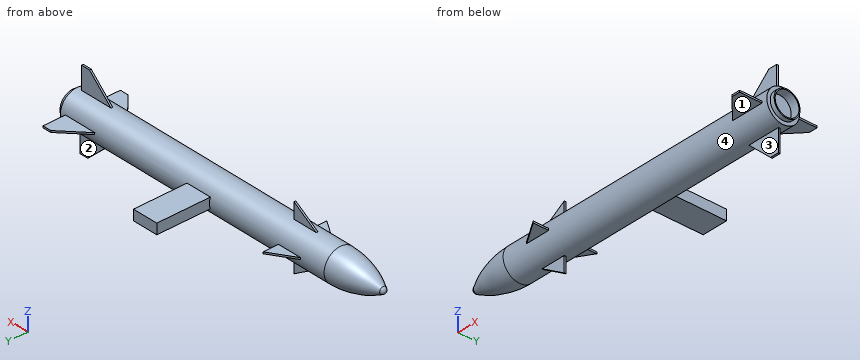
from build123d import *

# Parameters (mm, degrees)
D_ME1_FACE_RADIUS            = 400
D_ME1_HEIGHT                 = 290
ESQUISSE2_R                  = 1377.564968988
ENL_V_MAT_EXTRU_1_DEPTH      = 1000
BOSS_EXTRU_1_DEPTH           = 200
R_P_TITION_CIRCULAIRE1_COUNT = 4
BOSS_EXTRU_2_DEPTH           = 100
R_P_TITION_CIRCULAIRE2_COUNT = 4
ESQUISSE6_W                  = 3000
ESQUISSE6_H                  = 1200
BOSS_EXTRU_3_DEPTH           = 8000
ECHELLE1_SCALE               = 0.05


with BuildPart() as part:
    # Esquisse1 → Révolution1 (revolve)
    with BuildSketch(Plane(origin=(0, 0, 0), x_dir=(1, 0, 0), z_dir=(0, 1, 0))):
        with BuildLine():
            Line((0, 0), (0, 400))
            ThreePointArc((0, 400), (2649.561437252, 1518.274730075), (5500, 1900))
            Line((5500, 1900), (39500, 1900))
            Line((39500, 1900), (39500, 1500))
            Line((39500, 1500), (40000, 1500))
            Line((40000, 1500), (40000, 0))
            Line((40000, 0), (0, 0))
        make_face()
    revolve(axis=Axis((40000, 0, 0), (-1, 0, 0)))

    # Dôme1: a dome of height H over a round flat face of radius A is a cap of a sphere of radius (A * A + H * H) / (2 * H)
    d_me1_r = (D_ME1_FACE_RADIUS * D_ME1_FACE_RADIUS + D_ME1_HEIGHT * D_ME1_HEIGHT) / (2 * D_ME1_HEIGHT)
    d_me1_base = Plane((0, 0, 0), z_dir=(-1, 0, 0))
    with Locations(d_me1_base.offset(D_ME1_HEIGHT - d_me1_r)):
        d_me1_ball = Sphere(d_me1_r, mode=Mode.PRIVATE)
    add(split(d_me1_ball, bisect_by=d_me1_base, keep=Keep.TOP, mode=Mode.PRIVATE))

    # Esquisse2 → Enlèv. mat.-Extru.1 (cut)
    with BuildSketch(Plane(origin=(40000, 0, 0), x_dir=(0, 0, -1), z_dir=(1, 0, 0))):
        Circle(ESQUISSE2_R)
    extrude(amount=-ENL_V_MAT_EXTRU_1_DEPTH, mode=Mode.SUBTRACT)

    # Esquisse3 → Boss.-Extru.1 (add)
    with BuildSketch(Plane.XY):
        Polygon((38867.882175008, 1693.755150427), (38867.882175008, 4480.75805387), (37867.882175008, 4480.75805387), (34867.882175008, 1693.755150427), align=None)
    boss_extru_1 = extrude(amount=BOSS_EXTRU_1_DEPTH)

    # Répétition circulaire1: Boss.-Extru.1 ×4 about axis
    r_p_tition_circulaire1_axis = Axis((0, 0, 0), (1, 0, 0))
    for i in range(1, R_P_TITION_CIRCULAIRE1_COUNT):
        add(boss_extru_1.rotate(r_p_tition_circulaire1_axis, i * 360 / R_P_TITION_CIRCULAIRE1_COUNT))

    # Esquisse4 → Boss.-Extru.2 (add, symmetric)
    with BuildSketch(Plane.XY):
        Polygon((8155.279549148, 1665.288677311), (11371.991011305, 3686.408268577), (11371.991011305, 1665.288677311), align=None)
    boss_extru_2 = extrude(amount=BOSS_EXTRU_2_DEPTH, both=True)

    # Répétition circulaire2: Boss.-Extru.2 ×4 about axis
    r_p_tition_circulaire2_axis = Axis((0, 0, 0), (1, 0, 0))
    for i in range(1, R_P_TITION_CIRCULAIRE2_COUNT):
        add(boss_extru_2.rotate(r_p_tition_circulaire2_axis, i * 360 / R_P_TITION_CIRCULAIRE2_COUNT))

    # Esquisse6 → Boss.-Extru.3 (add)
    with BuildSketch(Plane(origin=(0, 0, 0), x_dir=(1, 0, 0), z_dir=(0, 1, 0))):
        with Locations((21779.89327035, -36.087335649)):
            Rectangle(ESQUISSE6_W, ESQUISSE6_H)
    extrude(amount=BOSS_EXTRU_3_DEPTH)


with BuildPart() as part_1:
    # Echelle1: scaled about (20884.167787821, 241.899239244, 1.78815963)
    add(part.part.scale(ECHELLE1_SCALE).moved(Location((19839.95939843, 229.804277282, 1.698751648))))


solid = part_1.part
Can you work these out from the model? Positions are in its coordinate system, mm. Face numbers are marked on the shaded views. A direction names the side the tool comes from. Give positions to 0.01 mm unless a question says otherwise; leave off trailing zeros. Loops run counter-clockwise (first coordinate to the right, second up) from the corner with the lowest first, then second, coordinate; pieces in that order, holes last. Notation, with made-up numbers: (16.25, 0.25) -> (55.25, 0.25) arc R11 ccw to (55.25, 13.25) -> close; hole circle Ø3 at (86, 11.25). An arc over 180 degrees is marked (long way). Return JSON: item names as keys, results as strings.
Q1. I want a section at A-A, the plane z = 145. List the corners of the cut face in (x, y) for me.
Checks:
{"outline": "(20343.27, 224.8) -> (20408.56, 224.8) -> (20408.56, 234.8) -> (20343.27, 234.8) -> close; (21646.45, 219.8) -> (21783.35, 219.8) -> (21783.35, 229.8) -> (21646.45, 229.8) -> close"}
Q2. For pin 1 Ø8 at (y, z) = (229.5, -133.5) entering from +X; pin 2 Ø3 at (y, z) = (351, -0.5) entering from +X; pin 3 Ø3 at (x, z) = (20147, 50.5) entering from +Y, each with a flat end and sliding along its axis, tell me the tip position at first contact or that it passes through.
Checks:
{"pin 1": "stops at x = 21783.35", "pin 2": "stops at x = 21003.95", "pin 3": "stops at y = 312.19"}
Q3. I want a section at B-B, the plane y = 79.5. List the corners of the cut face in (x, z) for me.
Checks:
{"outline": "(20354.42, -3.3) -> (20408.56, -3.3) -> (20408.56, 6.7) -> (20354.42, 6.7) -> close; (21653.98, -8.3) -> (21783.35, -8.3) -> (21783.35, 1.7) -> (21653.98, 1.7) -> close"}
Q4. I want a section at D-D, the plane y = 539.5. List the corners of the cut face in (x, z) for me, then the cut area to 3 significant figures.
Checks:
{"outline": "(20853.95, -26.5) -> (21003.95, -26.5) -> (21003.95, 33.5) -> (20853.95, 33.5) -> close", "area": "9,000 mm2"}
Q5. On a 3-axis mill with a long thin cutter (end or side, diameter ignored), from which of +Z, -Z, +X, -X, +Y, -Y can I reach the whole of each face in a straight line? I mean the marked faces 1, 2, 3 and 4. Say none if no direction works.
Checks:
{"face 1": "-Z, +X, -X, -Y", "face 2": "-Z, +X, -X, +Y", "face 3": "-Z, +X, -Y", "face 4": "none"}
Q6. I want a section at C-C, the plane x = 21709.5. List the corners of the cut face in (y, z) for me.
Checks:
{"outline": "(27.93, -8.3) -> (135.33, -8.3) arc R95 ccw to (229.8, -93.3) -> (229.8, -200.18) -> (239.8, -200.18) -> (239.8, -92.77) arc R95 ccw to (324.8, 1.7) -> (431.68, 1.7) -> (431.68, 11.7) -> (324.28, 11.7) arc R95 ccw to (229.8, 96.7) -> (229.8, 203.58) -> (219.8, 203.58) -> (219.8, 96.17) arc R95 ccw to (134.8, 1.7) -> (27.93, 1.7) -> close"}
Q7. I need wall thicknesses on probe 1 along Y at (x, z) = (21493.5, 8.5); probe 2 along Z at (x, y) = (20966, 323); probe 3 along Y at (x, z) = (21286.5, 0.5). Which ranges of each line are inside material? Lowest first, please.
Checks:
{"probe 1": "y = 135.05 to 324.56", "probe 2": "z = -26.5 to 33.5", "probe 3": "y = 134.81 to 324.8"}
